Check sheet for the modelled part. Datum: model origin and axes. Units: mm. Face numbers are marked on the shaded views. A direction names the side the tool comes from. Round coordinates to 2 decimals unless told otherwise and drop trailing zeros. Order: outer loops, then holes, each group sorted by start corner. A loop starts at its lowest first (then second) coordinate and runs counter-clockwise, first axis right, second up.
(1) Tool access check on the marked faces 1 and 2. Record the directions out of +Z, -Z, +X, -X, +Y, -Y that give a thin tool (end or side, any length) a straight path to the whole face; none if there is none.
(2) Sectioned sample at C-C, the plane z = 21. Enter the section's corners in (x, y).
(3) Sectioned sample at B-B, the plane y = 188.5. Enter the section's corners in (x, z), and give its area (3 significant figures).
(4) Sectioned sample at D-D, the plane y = 216. Enter the section's corners in (x, z), and give its area (3 significant figures).
(5) Sectioned sample at A-A, the plane x = 0. Enter the section's corners in (y, z), and give its area (3 significant figures).
(6) Depth check by flat-ended pin: pin 1 (6.5 mm diameter, centred on y = 249.27, z = 0, fed in from -X); pin 2 (3 mm diameter, centred on y = 72.5, z = -8.5, fed in from -X); pin 3 (6 mm diameter, centred on x = -9, z = 13.5, fed in from +Y); pin 4 (3 mm diameter, centred on x = -11.5, y = 116, fed in from +Z). Enter the tip coordinate at first touch or a pass-through.
(7) Thickness scan on probe 1 along X at (y, z) = (14.5, -1); probe 2 along Y at (x, z) = (13.5, 1.5); probe 3 along Z at (x, y) = (-0.5, 226). Record the ranges inside material, lowest first.
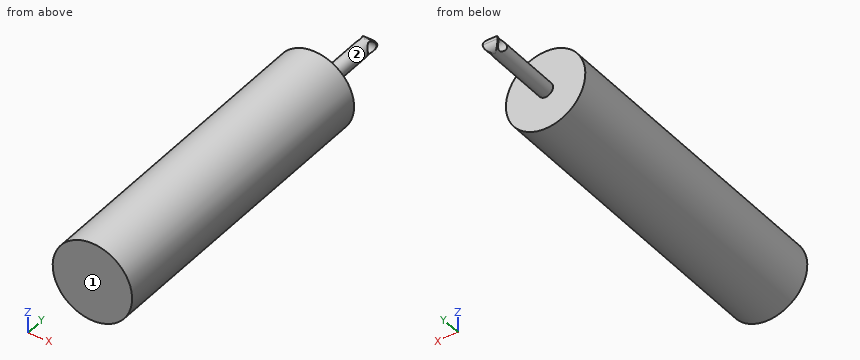
```python
from build123d import *

# Parameters (mm, degrees)
SKETCH1_R               = 25.4
BOSS_EXTRUDE1_DEPTH     = 203.2
SKETCH2_R               = 4.73075
BOSS_EXTRUDE2_DEPTH     = 50.8
CUT_EXTRUDE1_DEPTH      = 257.527425434
CUT_EXTRUDE1_DEPTH_BACK = 257.527425434
SKETCH3_R               = 3.96875


with BuildPart() as part:
    # Sketch1 → Boss-Extrude1 (new body)
    with BuildSketch(Plane(origin=(0, 0, 0), x_dir=(1, 0, 0), z_dir=(0, 1, 0))):
        with Locations(Location((0, 0, 0), (0, 0, 270))):
            Circle(SKETCH1_R)
    extrude(amount=BOSS_EXTRUDE1_DEPTH)

    # Sketch2 → Boss-Extrude2 (add)
    with BuildSketch(Plane(origin=(0, 203.2, 0), x_dir=(1, 0, 0), z_dir=(0, 1, 0))):
        with Locations(Location((0, 0, 0), (0, 0, 270))):
            Circle(SKETCH2_R)
    extrude(amount=BOSS_EXTRUDE2_DEPTH)

    # Sketch3 → Cut-Extrude1 (cut, two sides: drawn at the far end of the back side and taken through both)
    with BuildSketch(Plane(origin=(0, 0, 0), x_dir=(0, 0, -1), z_dir=(1, 0, 0)).offset(-CUT_EXTRUDE1_DEPTH_BACK)):
        with Locations((0, 249.26925)):
            Circle(SKETCH3_R)
        with BuildLine():
            Line((-4.73075, 254), (-4.73075, 249.26925))
            ThreePointArc((-4.73075, 249.26925), (-3.345145405, 252.614395405), (0, 254))
            Line((0, 254), (-4.73075, 254))
        make_face()
        with BuildLine():
            ThreePointArc((0, 254), (3.345145405, 252.614395405), (4.73075, 249.26925))
            Line((4.73075, 249.26925), (4.73075, 254))
            Line((4.73075, 254), (0, 254))
        make_face()
    extrude(amount=CUT_EXTRUDE1_DEPTH + CUT_EXTRUDE1_DEPTH_BACK, mode=Mode.SUBTRACT)


solid = part.part
```
Derived:
1. face 1: +Z, -Z, +X, -X, -Y
1. face 2: +Y
2. outline: (-14.29, 0) - (14.29, 0) - (14.29, 203.2) - (-14.29, 203.2) - close
3. outline: circle Ø50.8 at (0, 0)
3. area: 2,030 mm2
4. outline: circle Ø9.46 at (0, 0)
4. area: 70.3 mm2
5. outline: (0, -25.4) - (203.2, -25.4) - (203.2, -4.73) - (249.27, -4.73) arc R4.73 ccw to (249.27, 4.73) - (203.2, 4.73) - (203.2, 25.4) - (0, 25.4) - close; hole circle Ø7.94 at (249.27, 0)
5. area: 10,700 mm2
6. pin 1: passes through
6. pin 2: stops at x = -24.42
6. pin 3: stops at y = 203.2
6. pin 4: stops at z = 23.35
7. probe 1: x = -25.38 to 25.38
7. probe 2: y = 0 to 203.2
7. probe 3: z = -4.7 to 4.7
